```python
from build123d import *

# Parameters (mm, degrees)
SKETCH1_W           = 83
SKETCH1_H           = 79
BOSS_EXTRUDE1_DEPTH = 10.5
SHELL1_T            = 4
SKETCH4_W           = 53
SKETCH4_H           = 19
BOSS_EXTRUDE2_DEPTH = 26
SKETCH5_W           = 22
SKETCH5_H           = 45
CUT_EXTRUDE1_DEPTH  = 15
SKETCH7_W           = 8
SKETCH7_H           = 3
CUT_EXTRUDE2_DEPTH  = 4
SKETCH8_W           = 10
SKETCH8_H           = 10
CUT_EXTRUDE3_DEPTH  = 4
SKETCH9_W           = 53
SKETCH9_H           = 3
BOSS_EXTRUDE4_DEPTH = 10
SKETCH10_W          = 87
SKETCH10_H          = 3
BOSS_EXTRUDE5_DEPTH = 10
SKETCH11_W          = 7
SKETCH11_H          = 47
SKETCH11_H_2        = 81
CUT_EXTRUDE4_DEPTH  = 3
SKETCH12_W          = 10
SKETCH12_H          = 16
CUT_EXTRUDE5_DEPTH  = 4


with BuildPart() as part:
    # Sketch1 → Boss-Extrude1 (new, symmetric)
    with BuildSketch(Plane(origin=(0, 0, 0), x_dir=(1, 0, 0), z_dir=(0, 1, 0))):
        Rectangle(SKETCH1_W, SKETCH1_H)
    extrude(amount=BOSS_EXTRUDE1_DEPTH, both=True)

    # Shell1
    shell1_openings = [part.faces().sort_by_distance(p)[0] for p in [
        (0, 10.5, 0),
    ]]
    offset(amount=SHELL1_T, openings=shell1_openings, kind=Kind.INTERSECTION)

    # Sketch4 → Boss-Extrude2 (add)
    with BuildSketch(Plane(origin=(45.5, 0, 0), x_dir=(0, 0, -1), z_dir=(1, 0, 0))):
        with Locations((0, -5)):
            Rectangle(SKETCH4_W, SKETCH4_H)
    extrude(amount=BOSS_EXTRUDE2_DEPTH)

    # Sketch5 → Cut-Extrude1 (cut)
    with BuildSketch(Plane(origin=(0, 4.5, 0), x_dir=(1, 0, 0), z_dir=(0, 1, 0))):
        with Locations((56.5, 0)):
            Rectangle(SKETCH5_W, SKETCH5_H)
    extrude(amount=-CUT_EXTRUDE1_DEPTH, mode=Mode.SUBTRACT)

    # Sketch7 → Cut-Extrude2 (cut)
    with BuildSketch(Plane(origin=(0, 0, 22.5), x_dir=(-1, 0, 0), z_dir=(0, 0, -1))):
        with Locations((-54, -3)):
            Rectangle(SKETCH7_W, SKETCH7_H)
    extrude(amount=-CUT_EXTRUDE2_DEPTH, mode=Mode.SUBTRACT)

    # Sketch8 → Cut-Extrude3 (cut)
    with BuildSketch(Plane.XY.offset(-22.5)):
        with Locations((59.5, -0.5)):
            Rectangle(SKETCH8_W, SKETCH8_H)
    extrude(amount=-CUT_EXTRUDE3_DEPTH, mode=Mode.SUBTRACT)

    # Sketch9 → Boss-Extrude4 (add)
    with BuildSketch(Plane(origin=(71.5, 0, 0), x_dir=(0, 0, -1), z_dir=(1, 0, 0))):
        with Locations((0, -13)):
            Rectangle(SKETCH9_W, SKETCH9_H)
    extrude(amount=BOSS_EXTRUDE4_DEPTH)

    # Sketch10 → Boss-Extrude5 (add)
    with BuildSketch(Plane.ZY.offset(45.5)):
        with Locations((0, -13)):
            Rectangle(SKETCH10_W, SKETCH10_H)
    extrude(amount=BOSS_EXTRUDE5_DEPTH)

    # Sketch11 → Cut-Extrude4 (cut)
    with BuildSketch(Plane(origin=(0, -11.5, 0), x_dir=(1, 0, 0), z_dir=(0, 1, 0))):
        with Locations((75, 0)):
            Rectangle(SKETCH11_W, SKETCH11_H)
        with Locations((-49, 0)):
            Rectangle(SKETCH11_W, SKETCH11_H_2)
    extrude(amount=-CUT_EXTRUDE4_DEPTH, mode=Mode.SUBTRACT)

    # Sketch12 → Cut-Extrude5 (cut)
    with BuildSketch(Plane(origin=(45.5, 0, 0), x_dir=(0, 0, -1), z_dir=(1, 0, 0))):
        with Locations((14.5, 2.5)):
            Rectangle(SKETCH12_W, SKETCH12_H)
    extrude(amount=-CUT_EXTRUDE5_DEPTH, mode=Mode.SUBTRACT)


solid = part.part
```
Input: part model. Units: mm. Frame: model coordinates. A direction names the side the tool comes from. Round coordinates to 2 decimals unless told otherwise and drop trailing zeros. Order: outer loops, then holes, each group sorted by start corner. A loop starts at its lowest first (then second) coordinate and runs counter-clockwise, first axis right, second up. Notation, with made-up numbers: (-21, 74) - (28, 74) arc R9 ccw to (28, 86) - close; hole circle Ø11 at (-24.75, -33). An arc over 180 degrees is marked (long way). Answer in a Markdown table with one row per item.
Item 1: Section query C-C (z = -30). Return the cut outline in (x, y), then the cut area to 3 significant figures.
Model answer:
| item | result |
|---|---|
| outline | (-55.5, -14.5) - (-52.5, -14.5) - (-52.5, -11.5) - (-55.5, -11.5) - close; (-45.5, -14.5) - (45.5, -14.5) - (45.5, 10.5) - (41.5, 10.5) - (41.5, -10.5) - (-41.5, -10.5) - (-41.5, 10.5) - (-45.5, 10.5) - close |
| area | 541 mm² |
Item 2: Section query B-B (x = 52). Return the cut outline in (y, z), then the cut area to 3 significant figures.
Model answer:
| item | result |
|---|---|
| outline | (-14.5, -26.5) - (4.5, -26.5) - (4.5, -22.5) - (-10.5, -22.5) - (-10.5, 22.5) - (-4.5, 22.5) - (-4.5, 26.5) - (-14.5, 26.5) - close; (-1.5, 22.5) - (4.5, 22.5) - (4.5, 26.5) - (-1.5, 26.5) - close |
| area | 320 mm² |
Item 3: Section query D-D (y = -8). Return the cut outline in (x, z), then the cut area to 3 significant figures.
Model answer:
| item | result |
|---|---|
| outline | (-45.5, -43.5) - (45.5, -43.5) - (45.5, -26.5) - (71.5, -26.5) - (71.5, 26.5) - (45.5, 26.5) - (45.5, 43.5) - (-45.5, 43.5) - close; hole (-41.5, -39.5) - (41.5, -39.5) - (41.5, 39.5) - (-41.5, 39.5) - close; hole (45.5, -22.5) - (67.5, -22.5) - (67.5, 22.5) - (45.5, 22.5) - close |
| area | 1,750 mm² |
Item 4: Section query A-A (z = 0.5). Return the cut outline in (x, y).
Model answer:
| item | result |
|---|---|
| outline | (-55.5, -14.5) - (-52.5, -14.5) - (-52.5, -11.5) - (-55.5, -11.5) - close; (-45.5, -14.5) - (71.5, -14.5) - (71.5, 4.5) - (67.5, 4.5) - (67.5, -10.5) - (45.5, -10.5) - (45.5, 10.5) - (41.5, 10.5) - (41.5, -10.5) - (-41.5, -10.5) - (-41.5, 10.5) - (-45.5, 10.5) - close; (78.5, -14.5) - (81.5, -14.5) - (81.5, -11.5) - (78.5, -11.5) - close |
Item 5: Pin query (flat end, axial travel): pin 1 (24 mm diameter, centred on x = 61.5, z = -5, fed in from +Y); pin 2 (2.5 mm diameter, centred on y = -2.5, z = 25, fed in from -X); pin 3 (15 mm diameter, centred on x = 60, y = -5, fed in from +Z). Return the tip coordinate at first contact, or that it passes through.
Model answer:
| item | result |
|---|---|
| pin 1 | stops at y = 4.5 |
| pin 2 | stops at x = -45.5 |
| pin 3 | stops at z = 26.5 |
Item 6: Reachability of faces 1 (the flat face through (75, -13, 23.5)), 2 (the flat face through (79, -11.5, 6)), 3 (the flat face through (54, -4.5, 24)), 4 (the flat face through (56, -10.5, 0)), 5 (the flat face through (54.5, -1, -24)) from +Z, -Z, +X, -X, +Y, -Y: full face, straight path, thin tool, end or side. Return the list, or none.
Model answer:
| item | result |
|---|---|
| face 1 | +Y, -Y |
| face 2 | +Z, -Z, +X, +Y |
| face 3 | +Z |
| face 4 | +Y |
| face 5 | -Z, +Y |
Item 7: Line query: line 1 (X direction, y = 3, z = -1); line 2 (X direction, y = -5.25, z = 25); line 3 (Z direction, x = 11, y = 4.25). Output: solid intervals per line, ascending.
Model answer:
| item | result |
|---|---|
| line 1 | x = -45.5 to -41.5, 41.5 to 45.5, 67.5 to 71.5 |
| line 2 | x = -45.5 to -41.5, 41.5 to 71.5 |
| line 3 | z = -43.5 to -39.5, 39.5 to 43.5 |
Item 8: Mould query, pull axis Z, two halves, no side actions, for faces 6 (the flat face through (78.5, -13, 0)), 7 (the flat face through (58, -3, 24)), 8 (the flat face through (59, -7, -26.5)). Classes: released by +Z, released by -Z, zero draft, split by the parting line, or undercut.
Model answer:
| item | result |
|---|---|
| face 6 | undercut |
| face 7 | zero draft |
| face 8 | released by -Z |
